```python
from build123d import *

# Parameters (mm, degrees)
BOSS_EXTRUDE1_DEPTH = 6.35
FILLET1_R           = 3.175


with BuildPart() as part:
    # Sketch2 → Boss-Extrude1 (new body)
    with BuildSketch(Plane.XY):
        Polygon((25.4, 65.0875), (58.7375, 65.0875), (58.7375, -65.0875), (-58.7375, -65.0875), (-58.7375, 65.0875), (-25.4, 65.0875), (-25.4, 71.4375), (25.4, 71.4375), align=None)
    extrude(amount=BOSS_EXTRUDE1_DEPTH)

    # Fillet1
    fillet1_edges = [part.edges().sort_by_distance(p)[0] for p in [
        (-58.7375, -65.0875, 3.175),
        (58.7375, -65.0875, 3.175),
        (58.7375, 65.0875, 3.175),
        (-58.7375, 65.0875, 3.175),
    ]]
    fillet(fillet1_edges, radius=FILLET1_R)


solid = part.part
```
Input: part model. Units: mm. Frame: model coordinates. A direction names the side the tool comes from. Coordinates: 2 decimals unless noted, no trailing zeros. Write each loop counter-clockwise with the first axis right and the second up, starting at its lowest first coordinate (ties: lowest second). Pieces come first, ordered by that corner, then holes.
1) Pin query (flat end, axial travel): pin 1 Ø1.5 at (x, z) = (36.5, 3) entering from +Y; pin 2 Ø1.9 at (y, z) = (67, 3.5) entering from +X. Return the tip coordinate at first contact, or that it passes through.
2) Set-up query: faces 1 (the cylindrical face through (-57.783, -64.182, 3.219)), 2 (the flat face through (40, 65.088, 3)), 3 (the flat face through (-25.4, 68, 3)). Return all of +Z, -Z, +X, -X, +Y, -Y with unobstructed straight access to the full face (end or side cutting, diameter ignored); none if empty.
3) Section B-B on x = -42. Output: boundary loops of the cut face in (y, z).
4) Mould query, pull axis Y, two halves, no side actions, for faces 4 (the cylindrical face through (-57.832, 64.133, 3.219)), 5 (the flat face through (25.4, 68, 3)), 6 (the flat face through (1, -65.088, 3)). Classes: pulls with the +Y half, pulls with the -Y half, needs draft (parallel to the pull), parting line crosses it, or undercut.
5) Material intervals for line 1 along Y through (x, z) = (-46, 4), sorted ascending.
Check result:
1. pin 1: stops at y = 65.09
1. pin 2: stops at x = 25.4
2. face 1: +Z, -Z, -X, -Y
2. face 2: +Z, -Z, +X, +Y
2. face 3: +Z, -Z, -X, +Y
3. outline: (-65.09, 0) - (65.09, 0) - (65.09, 6.35) - (-65.09, 6.35) - close
4. face 4: pulls with the +Y half
4. face 5: needs draft
4. face 6: pulls with the -Y half
5. line 1: y = -65.09 to 65.09
